The model under review builds one solid part; all positions refer to its coordinate system, in mm. Face numbers are marked on the shaded views. Give positions to 0.01 mm unless a question says otherwise; leave off trailing zeros. Write each loop counter-clockwise with the first axis right and the second up, starting at its lowest first coordinate (ties: lowest second). Pieces come first, ordered by that corner, then holes. Notation, with made-up numbers: M -26.5,41 L -15.5,41 A5 ccw -15.5,46 Z; hole C -20.75,78.5 d2. An arc over 180 degrees is marked long. Write each question's results on one line, items separated by ' | '. Start each with the question number.
from build123d import *

# Parameters (mm, degrees)
MODEL_R                 = 8.05
SALIENTE_EXTRUIR1_DEPTH = 3
CROQUIS2_W              = 3
CROQUIS2_H              = 36.500000005
SALIENTE_EXTRUIR2_DEPTH = 18.8
REDONDEO1_R             = 2
CROQUIS3_R              = 0.75
CROQUIS3_W              = 11.8
CROQUIS3_H              = 22.5
CORTAR_EXTRUIR1_DEPTH   = 15.8
CROQUIS7_R              = 1.5
CORTAR_EXTRUIR3_DEPTH   = 1
SIMETR_A1_START         = 177.868163256
SIMETR_A1_OUTLINE_R     = 1.5
SIMETR_A1_OUTLINE_W     = 22.5
SIMETR_A1_OUTLINE_H     = 11.8
SIMETR_A1_DEPTH         = 3
SIMETR_A1_2_OUTLINE_R   = 1.5
SIMETR_A1_2_OUTLINE_R_2 = 0.75
SIMETR_A1_2_DEPTH       = 2
CROQUIS5_W              = 20
CROQUIS5_H              = 3
SALIENTE_EXTRUIR3_DEPTH = 11
REDONDEO2_R             = 2
CROQUIS6_R              = 1.289460228
CORTAR_EXTRUIR2_DEPTH   = 3
CROQUIS8_R              = 2.25
CORTAR_EXTRUIR4_DEPTH   = 1
REDONDEO3_R             = 2


# Read off the part's stored shape, not the designer's step: Simetría1
with BuildPart() as part:
    # Model → Saliente-Extruir1 (new body)
    with BuildSketch(Plane.XY):
        with BuildLine():
            Line((129.495355099, -134.938548449), (149.495355099, -134.938548449))
            Line((149.495355099, -134.938548449), (149.495355099, -133.938548449))
            ThreePointArc((149.495355099, -133.938548449), (150.081141537, -132.524334887), (151.495355099, -131.938548449))
            Line((151.495355099, -131.938548449), (176.128197203, -131.938548449))
            ThreePointArc((176.128197203, -131.938548449), (177.538284884, -131.35687589), (178.128163256, -129.950201179))
            Line((178.128163256, -129.950201179), (177.862546943, -123.950201137))
            ThreePointArc((177.862546943, -123.950201137), (178.44833338, -122.535987575), (179.862546943, -121.950201137))
            Line((179.862546943, -121.950201137), (180.862546943, -121.950201137))
            Line((180.862546943, -121.950201137), (180.862546943, -85.450201132))
            Line((180.862546943, -85.450201132), (179.862546943, -85.450201132))
            ThreePointArc((179.862546943, -85.450201132), (178.44833338, -84.864414695), (177.862546943, -83.450201132))
            ThreePointArc((177.862546943, -83.450201132), (177.142837957, -82.533630305), (176.128163256, -81.960465095))
            ThreePointArc((176.128163256, -81.960465095), (166.435178179, -78.024818287), (159.872429316, -69.877818664))
            ThreePointArc((159.872429316, -69.877818664), (154.765410937, -73.462979643), (150.58174723, -78.092447642))
            ThreePointArc((150.58174723, -78.092447642), (144.486823712, -75.481596568), (140.942488903, -69.877818664))
            ThreePointArc((140.942488903, -69.877818664), (135.047590207, -72.161784577), (130.172970832, -76.18725559))
            ThreePointArc((130.172970832, -76.18725559), (127.440920733, -73.607562885), (126.984938003, -69.877818664))
            ThreePointArc((126.984938003, -69.877818664), (120.346137898, -72.294388425), (115.017340976, -76.933073543))
            ThreePointArc((115.017340976, -76.933073543), (113.269189628, -74.182373632), (113.071027177, -70.929203673))
            ThreePointArc((113.071027177, -70.929203673), (105.5068889, -74.040793408), (101.128163256, -80.949117392))
            Line((101.128163256, -80.949117392), (101.128163256, -83.450201132))
            ThreePointArc((101.128163256, -83.450201132), (100.542376818, -84.864414695), (99.128163256, -85.450201132))
            Line((99.128163256, -85.450201132), (98.128163256, -85.450201132))
            Line((98.128163256, -85.450201132), (98.128163256, -121.950201137))
            Line((98.128163256, -121.950201137), (99.128163256, -121.950201137))
            ThreePointArc((99.128163256, -121.950201137), (100.542376818, -122.535987575), (101.128163256, -123.950201137))
            Line((101.128163256, -123.950201137), (101.128163256, -129.950201137))
            ThreePointArc((101.128163256, -129.950201137), (101.714262231, -131.364727168), (103.129047148, -131.950200942))
            Line((103.129047148, -131.950200942), (127.494471207, -131.939432732))
            ThreePointArc((127.494471207, -131.939432732), (128.909256124, -132.524906506), (129.495355099, -133.939432537))
            Line((129.495355099, -133.939432537), (129.495355099, -134.938548449))
        make_face()
        with Locations((126.495355099, -99.894288355)):
            Circle(MODEL_R, mode=Mode.SUBTRACT)
        with Locations((152.495355099, -99.894288355)):
            Circle(MODEL_R, mode=Mode.SUBTRACT)
    extrude(amount=SALIENTE_EXTRUIR1_DEPTH)

    # Croquis2 → Saliente-Extruir2 (add)
    with BuildSketch(Plane.XY.offset(3)):
        with Locations((99.628163256, -103.700201135)):
            Rectangle(CROQUIS2_W, CROQUIS2_H)
    extrude(amount=-SALIENTE_EXTRUIR2_DEPTH)

    # Redondeo1
    redondeo1_edges = [part.edges().sort_by_distance(p)[0] for p in [
        (99.628163256, -121.950201137, -15.8),
        (99.628163256, -85.450201132, -15.8),
        (98.128163256, -103.700201135, 3),
    ]]
    fillet(redondeo1_edges, radius=REDONDEO1_R)

    # Croquis3 → Cortar-Extruir1 (cut)
    with BuildSketch(Plane.ZY.offset(-98.128163256)):
        with Locations((-7.9, -117.350201137)):
            Circle(CROQUIS3_R)
        with Locations((-7.9, -90.050201137)):
            Circle(CROQUIS3_R)
        with Locations((-7.9, -103.700201137)):
            Rectangle(CROQUIS3_W, CROQUIS3_H)
    extrude(amount=-CORTAR_EXTRUIR1_DEPTH, mode=Mode.SUBTRACT)

    # Croquis7 → Cortar-Extruir3 (cut)
    with BuildSketch(Plane.ZY.offset(-98.128163256)):
        with Locations((-7.9, -90.050201137)):
            Circle(CROQUIS7_R)
        with Locations((-7.9, -117.350201137)):
            Circle(CROQUIS7_R)
    extrude(amount=-CORTAR_EXTRUIR3_DEPTH, mode=Mode.SUBTRACT)

    # Simetría1 outline → Simetría1 (add)
    with BuildSketch(Plane.YZ.offset(SIMETR_A1_START)):
        with BuildLine():
            ThreePointArc((-121.950201137, -13.8), (-121.364414699, -15.214213562), (-119.950201137, -15.8))
            Line((-119.950201137, -15.8), (-87.450201132, -15.8))
            ThreePointArc((-87.450201132, -15.8), (-86.03598757, -15.214213562), (-85.450201132, -13.8))
            Line((-85.450201132, -13.8), (-85.450201132, 3))
            Line((-85.450201132, 3), (-121.950201137, 3))
            Line((-121.950201137, 3), (-121.950201137, -13.8))
        make_face()
        with Locations((-117.350201137, -7.9)):
            Circle(SIMETR_A1_OUTLINE_R, mode=Mode.SUBTRACT)
        with Locations((-103.700201137, -7.9)):
            Rectangle(SIMETR_A1_OUTLINE_W, SIMETR_A1_OUTLINE_H, mode=Mode.SUBTRACT)
        with Locations((-90.050201137, -7.9)):
            Circle(SIMETR_A1_OUTLINE_R, mode=Mode.SUBTRACT)
    extrude(amount=SIMETR_A1_DEPTH)

    # Simetr_a1 2 outline → Simetr_a1 2 (add)
    # profile 1 of 2: a face of its own
    with BuildSketch(Plane.YZ.offset(SIMETR_A1_START)):
        with Locations((-117.350201137, -7.9)):
            Circle(SIMETR_A1_2_OUTLINE_R)
        with Locations((-117.350201137, -7.9)):
            Circle(SIMETR_A1_2_OUTLINE_R_2, mode=Mode.SUBTRACT)
    # profile 2 of 2: a face of its own
    with BuildSketch(Plane.YZ.offset(SIMETR_A1_START)):
        with Locations((-90.050201137, -7.9)):
            Circle(SIMETR_A1_2_OUTLINE_R)
        with Locations((-90.050201137, -7.9)):
            Circle(SIMETR_A1_2_OUTLINE_R_2, mode=Mode.SUBTRACT)
    extrude(amount=SIMETR_A1_2_DEPTH)

    # Croquis5 → Saliente-Extruir3 (add)
    with BuildSketch(Plane.XY.offset(3)):
        with Locations((139.495355099, -133.438548449)):
            Rectangle(CROQUIS5_W, CROQUIS5_H)
    extrude(amount=-SALIENTE_EXTRUIR3_DEPTH)

    # Redondeo2
    redondeo2_edges = [part.edges().sort_by_distance(p)[0] for p in [
        (129.495355099, -133.438548449, -8),
        (149.495355099, -133.438548449, -8),
    ]]
    fillet(redondeo2_edges, radius=REDONDEO2_R)

    # Croquis6 → Cortar-Extruir2 (cut)
    with BuildSketch(Plane(origin=(0, -131.938548449, 0), x_dir=(1, 0, 0), z_dir=(0, 1, 0))):
        with Locations(Location((133.495355099, 3.5, 0), (0, 0, 270))):
            Circle(CROQUIS6_R)
        with Locations(Location((145.495355099, 3.5, 0), (0, 0, 90))):
            Circle(CROQUIS6_R)
    extrude(amount=-CORTAR_EXTRUIR2_DEPTH, mode=Mode.SUBTRACT)

    # Croquis8 → Cortar-Extruir4 (cut)
    with BuildSketch(Plane(origin=(0, -131.938548449, 0), x_dir=(1, 0, 0), z_dir=(0, 1, 0))):
        with Locations(Location((145.495355099, 3.5, 0), (0, 0, 270))):
            Circle(CROQUIS8_R)
        with Locations(Location((133.495355099, 3.5, 0), (0, 0, 270))):
            Circle(CROQUIS8_R)
    extrude(amount=-CORTAR_EXTRUIR4_DEPTH, mode=Mode.SUBTRACT)

    # Redondeo3
    # the kernel refuses this fillet: 2 mm, written as the material it takes off along each edge
    with BuildSketch(Plane(origin=(180.868163256, -80.450201132, 3), x_dir=(-1, 0, 0), z_dir=(0, -1, 0))) as redondeo3_piece_1:
        with BuildLine():
            CenterArc((REDONDEO3_R, REDONDEO3_R), REDONDEO3_R, 180, 90)
            Line((0, REDONDEO3_R), (0, 0))
            Line((0, 0), (REDONDEO3_R, 0))
        make_face()
    extrude(amount=46.500000005, mode=Mode.SUBTRACT)


solid = part.part
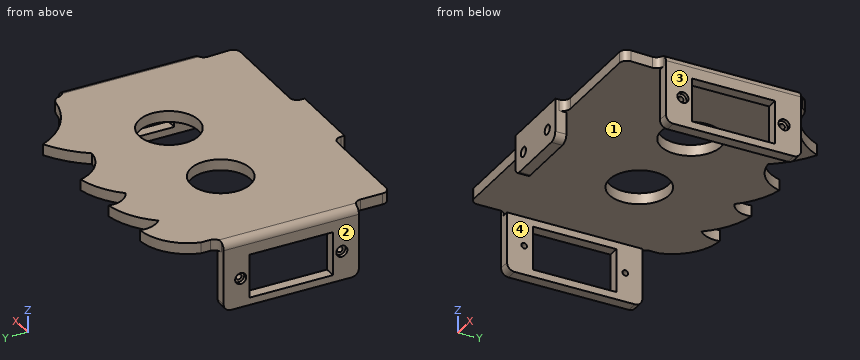
(1) Add section B-B (x = 156). State the section outline as (y, z) points.
(2) Add section D-D (z = -3.5). Give the number of separate pieces and of enclosed holes in the cut face, then the cut area to 3 significant figures.
(3) Clearance check with flat-ended pins moving along their axes: P1, Ø1.5, axis at x = 180, z = -3.5, coming from the +Y side; P2, Ø3.5, axis at y = -125.5, z = 1, coming from the -X side; P3, Ø4, axis at x = 145.5, z = -3.5, coming from the +Y side; P4, Ø1.5, axis at y = -113.5, z = -9.5, coming from the -X side. State where each tip first meets the part, or that it passes through.
(4) Add section C-C (y = -94). State the section outline as (x, z) points, then the cut area to 3 significant figures.
(5) Add section A-A (y = -113.5). State the section outline as (x, z) points.
(6) Draft analysis for pull direction X (two halves, no side actions). For the marked faces 1, 2, 3 and 4, state which applies: pulls with the +X half, pulls with the -X half, needs draft (parallel to the pull), parting line crosses it, or undercut.
(7) Wall thickness on L1, parallel to Y at x = 98.6, z = -7.9; L2, parallel to X at y = -132.2, z = -3.5; L3, parallel to X at y = -133.4, z = -3.5: over which ranges is each line inside the solid? List them lowest first.
Calculated:
1) outline: M -131.94,0 L -107.14,0 L -107.14,3 L -131.94,3 Z; M -92.65,0 L -72.43,0 L -72.43,3 L -92.65,3 Z
2) separate pieces: 7 | enclosed holes: 0 | area: 125 mm²
3) P1: stops at y = -85.45 | P2: stops at x = 101.12 | P3: stops at y = -132.94 | P4: passes through
4) outline: M 98.13,-15.8 L 101.13,-15.8 L 101.13,-13.8 L 98.13,-13.8 Z; M 98.13,-2 L 101.13,-2 L 101.13,0 L 121.01,0 L 121.01,3 L 100.13,3 A2 ccw 98.13,1 Z; M 131.98,0 L 147.01,0 L 147.01,3 L 131.98,3 Z; M 157.98,0 L 177.87,0 L 177.87,-2 L 180.87,-2 L 180.87,1 A2 ccw 178.87,3 L 157.98,3 Z; M 177.87,-15.8 L 180.87,-15.8 L 180.87,-13.8 L 177.87,-13.8 Z | area: 205 mm²
5) outline: M 98.13,-15.8 L 101.13,-15.8 L 101.13,-13.8 L 98.13,-13.8 Z; M 98.13,-2 L 101.13,-2 L 101.13,0 L 177.87,0 L 177.87,-2 L 180.87,-2 L 180.87,1 A2 ccw 178.87,3 L 100.13,3 A2 ccw 98.13,1 Z; M 177.87,-15.8 L 180.87,-15.8 L 180.87,-13.8 L 177.87,-13.8 Z
6) face 1: undercut | face 2: pulls with the -X half | face 3: pulls with the +X half | face 4: undercut
7) L1: y = -121.95 to -118.85, -115.85 to -114.95, -92.45 to -91.55, -88.55 to -85.45 | L2: x = 129.5 to 131.25, 135.75 to 143.25, 147.75 to 149.5 | L3: x = 129.5 to 132.21, 134.78 to 144.21, 146.78 to 149.5
